Check sheet for the modelled part. Datum: model origin and axes. Units: mm. Coordinates: 2 decimals unless noted, no trailing zeros. Loops run counter-clockwise (first coordinate to the right, second up) from the corner with the lowest first, then second, coordinate; pieces in that order, holes last. Notation, with made-up numbers: M 62.25,61 L 109.25,61 A19 cw 109.25,92 Z; hole C 63.25,61 d2. An arc over 180 degrees is marked long. Use CSV: the item, a comma, the result in double quotes. Start each with the question number.
(1) Section check B-B on z = 8.5. Record the cut outline in (x, y).
(2) Scan lines: line 1 (Z direction, x = -6, y = -1); line 2 (X direction, y = -1.25, z = -29.5); line 3 (Z direction, x = 28, y = -7). Record each from-to range of solid material in increasing order.
(3) Section check A-A on x = 4. Record the cut outline in (y, z).
(4) Go/stop test with flat-tipped pins: pin 1 Ø2 at (x, y) = (33, -5.5) entering from -Z; pin 2 Ø3 at (x, y) = (-22.5, -2.5) entering from +Z; pin 3 Ø3 at (x, y) = (-5.5, -6) entering from +Z. Record where each tip stops, or that it passes through.
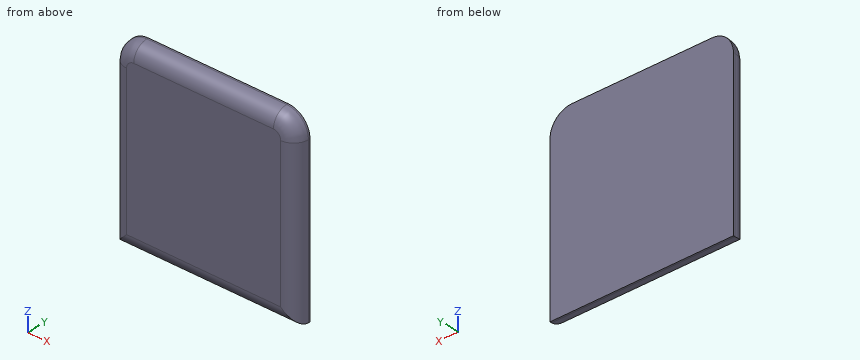
from build123d import *

# Parameters (mm, degrees)
F0_W        = 85.2935686707
F0_H        = 84.8211869597
F0_R        = 1.905
F0_R_2      = 0.8509
F1_DEPTH    = 7.62
F2_R        = 6.8125926862
F3_T1_DEPTH = 33.02
F3_T4_ANGLE = 90
F3_T6_ANGLE = 90


# Not quite as in the source:
# - a fillet or chamfer that OpenCascade refuses, or shapes differently, is made with other operations: its cross-section is extruded or revolved along the edge and cut away or added


with BuildPart() as f1:
    # F0 (on Front) → F1 (new body)
    with BuildSketch(Plane.XZ):
        Rectangle(F0_W, F0_H)
        Polygon((0, 38.1), (38.1, 38.1), (38.1, -38.1), (0, -38.1), (-38.1, -38.1), (-38.1, 38.1), align=None, mode=Mode.SUBTRACT)
        Polygon((25.4, 25.4), (0, 25.4), (-25.4, 25.4), (-25.4, -25.4), (0, -25.4), (25.4, -25.4), align=None)
        with Locations((-18.288, -12.446)):
            Circle(F0_R, mode=Mode.SUBTRACT)
        with Locations((19.812, -12.446)):
            Circle(F0_R, mode=Mode.SUBTRACT)
        with Locations((-18.288, 12.954)):
            Circle(F0_R, mode=Mode.SUBTRACT)
        with Locations((19.812, 12.954)):
            Circle(F0_R, mode=Mode.SUBTRACT)
        Polygon((0, 25.4), (0, 38.1), (-38.1, 38.1), (-38.1, -38.1), (0, -38.1), (0, -25.4), (-25.4, -25.4), (-25.4, 25.4), align=None)
        Polygon((38.1, -38.1), (38.1, 38.1), (0, 38.1), (0, 25.4), (25.4, 25.4), (25.4, -25.4), (0, -25.4), (0, -38.1), align=None)
        with Locations((-18.288, -12.446)):
            Circle(F0_R)
        with Locations((-18.288, -12.446)):
            Circle(F0_R_2, mode=Mode.SUBTRACT)
        with Locations((-18.288, 12.954)):
            Circle(F0_R)
        with Locations((-18.288, 12.954)):
            Circle(F0_R_2, mode=Mode.SUBTRACT)
        with Locations((19.812, 12.954)):
            Circle(F0_R)
        with Locations((19.812, 12.954)):
            Circle(F0_R_2, mode=Mode.SUBTRACT)
        with Locations((19.812, -12.446)):
            Circle(F0_R)
        with Locations((19.812, -12.446)):
            Circle(F0_R_2, mode=Mode.SUBTRACT)
        with Locations((-18.288, 12.954)):
            Circle(F0_R_2)
        with Locations((-18.288, -12.446)):
            Circle(F0_R_2)
        with Locations((19.812, 12.954)):
            Circle(F0_R_2)
        with Locations((19.812, -12.446)):
            Circle(F0_R_2)
    extrude(amount=F1_DEPTH)

    # F2
    f2_edges = [f1.edges().sort_by_distance(p)[0] for p in [
        (0, -7.62, -42.410593),
        (-42.646784, -7.62, 0),
        (0, -7.62, 42.410593),
        (42.646784, -7.62, 0),
    ]]
    fillet(f2_edges, radius=F2_R)

    # F3: fillet of radius 10.16 on 2 edges, made by hand

    # F3_s2 → F3_t1 (cut)
    with BuildSketch(Plane.XZ.offset(-25.4)):
        with BuildLine():
            ThreePointArc((42.6467843354, 32.2505934799), (39.6709892322, 39.4347983767), (32.4867843354, 42.4105934799))
            Line((32.4867843354, 42.4105934799), (42.6467843354, 42.4105934799))
            Line((42.6467843354, 42.4105934799), (42.6467843354, 32.2505934799))
        make_face()
        with BuildLine():
            ThreePointArc((-32.4867843354, 42.4105934799), (-39.6709892322, 39.4347983767), (-42.6467843354, 32.2505934799))
            Line((-42.6467843354, 32.2505934799), (-42.6467843354, 42.4105934799))
            Line((-42.6467843354, 42.4105934799), (-32.4867843354, 42.4105934799))
        make_face()
    extrude(amount=F3_T1_DEPTH, mode=Mode.SUBTRACT)

    # F3_s3 → F3_t4 (revolve, cut)
    with BuildSketch(Plane.YZ.offset(-32.4867843354)):
        with BuildLine():
            ThreePointArc((-7.62, 35.5980007937), (-5.6246377997, 40.4152312796), (-0.8074073138, 42.4105934799))
            Line((-0.8074073138, 42.4105934799), (-7.62, 42.4105934799))
            Line((-7.62, 42.4105934799), (-7.62, 35.5980007937))
        make_face()
    revolve(axis=Axis((-32.4867843354, -7.62, 32.2505934799), (0, -1, 0)), revolution_arc=F3_T4_ANGLE, mode=Mode.SUBTRACT)

    # F3_s5 → F3_t6 (revolve, cut)
    with BuildSketch(Plane.XY.offset(32.2505934799)):
        with BuildLine():
            ThreePointArc((35.8341916492, -7.62), (40.6514221351, -5.6246377997), (42.6467843354, -0.8074073138))
            Line((42.6467843354, -0.8074073138), (42.6467843354, -7.62))
            Line((42.6467843354, -7.62), (35.8341916492, -7.62))
        make_face()
    revolve(axis=Axis((32.4867843354, -7.62, 32.2505934799), (0, -1, 0)), revolution_arc=F3_T6_ANGLE, mode=Mode.SUBTRACT)


solid = f1.part
Outcome:
1,outline,"M -42.65,-0.81 A6.81 ccw -35.83,-7.62 L 35.83,-7.62 A6.81 ccw 42.65,-0.81 L 42.65,0 L -42.65,0 Z"
2,line 1,"z = -42.41 to 42.41"
2,line 2,"x = -42.63 to 42.63"
2,line 3,"z = -38.44 to 38.44"
3,outline,"M -7.62,-35.6 A6.81 ccw -0.81,-42.41 L 0,-42.41 L 0,42.41 L -0.81,42.41 A6.81 ccw -7.62,35.6 Z"
4,pin 1,"stops at z = -41.32"
4,pin 2,"stops at z = 42.41"
4,pin 3,"stops at z = 41.32"
